Study the drawing (mm; zero at the part's minimum x, y, z) and answer. A direction names the side the tool comes from. Round coordinates to 2 decimals unless told otherwise and drop trailing zeros. Write each loop counter-clockwise with the first axis right and the second up, starting at its lowest first coordinate (ties: lowest second). Pieces come first, ordered by that corner, then holes.
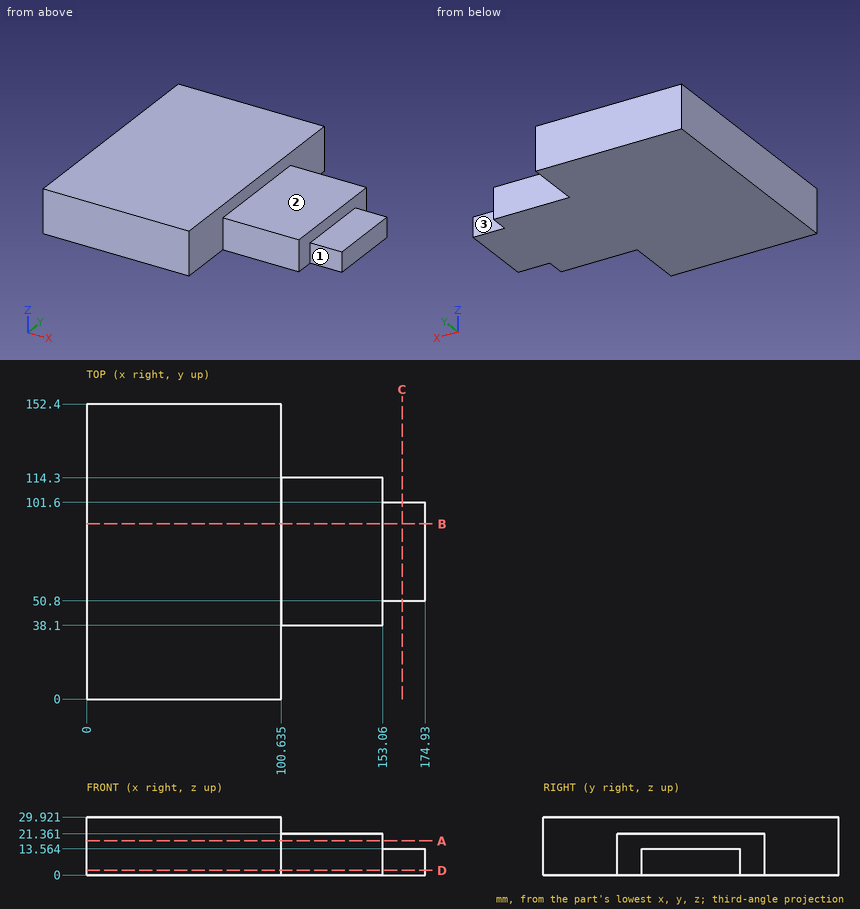
1. Section A-A on z = 17.75 is taken. Determine the outline of the cut face in (x, y) (1 decimal).
Geometry says:
outline: (0, 0) - (100.6, 0) - (100.6, 38.1) - (153.1, 38.1) - (153.1, 114.3) - (100.6, 114.3) - (100.6, 152.4) - (0, 152.4) - close
2. Section D-D on z = 2.5 is taken. Determine the outline of the cut face in (x, y) (1 decimal).
Geometry says:
outline: (0, 0) - (100.6, 0) - (100.6, 38.1) - (153.1, 38.1) - (153.1, 50.8) - (174.9, 50.8) - (174.9, 101.6) - (153.1, 101.6) - (153.1, 114.3) - (100.6, 114.3) - (100.6, 152.4) - (0, 152.4) - close
3. Section C-C on x = 163 is taken. Determine the outline of the cut face in (y, z), plus the area to 3 significant figures.
Geometry says:
outline: (50.8, 0) - (101.6, 0) - (101.6, 13.56) - (50.8, 13.56) - close
area: 689 mm2
4. A tool of negligible diameter and unlimited length cuts with its end or side. For the marked faces 1, 2 and 3, from which of +Z, -Z, +X, -X, +Y, -Y can it reach the whole face along a straight path? Write none if from no direction.
Geometry says:
face 1: +Z, -Z, +X, -Y
face 2: +Z, +X, +Y, -Y
face 3: +Z, -Z, +X, +Y
5. Straight lines are drawn through the part: line 1 along Z through (x, y) = (113, 111); line 2 along Y through (x, z) = (145, 4.75); line 3 along X through (y, z) = (111, 23.25) (1 decimal). For each, find the intervals that lie inside material, in ascending order.
Geometry says:
line 1: z = 0 to 21.36
line 2: y = 38.1 to 114.3
line 3: x = 0 to 100.6
6. Given pin 1 (6.5 mm diameter, centred on x = 133, z = 7, fed in from -Y); pin 2 (5 mm diameter, centred on y = 89, z = 25, fed in from +X) (1 decimal); pin 3 (11 mm diameter, centred on x = 166.5, y = 76, fed in from +Z); pin 4 (1 mm diameter, centred on y = 29.5, z = 9.5, fed in from -X), each flat-ended and moving along its own axis, determine where each tip first touches the part or whether it passes through.
Geometry says:
pin 1: stops at y = 38.1
pin 2: stops at x = 100.6
pin 3: stops at z = 13.56
pin 4: stops at x = 0
7. Section B-B on y = 90.5 is taken. Determine the outline of the cut face in (x, z) (1 decimal), plus the area to 3 significant figures.
Geometry says:
outline: (0, 0) - (174.9, 0) - (174.9, 13.6) - (153.1, 13.6) - (153.1, 21.4) - (100.6, 21.4) - (100.6, 29.9) - (0, 29.9) - close
area: 4,430 mm2
